Autodesk Inventor part; units mm, degrees
ref_plane "Work Plane3" through (158.3589, -41.348, 102.8428) normal (0, 0, -1) x (-1, 0, 0)
ref_plane "Work Plane5" through (0, -98.2767, 225.7428) normal (0, 1, 0) x (-1, 0, 0)
ref_plane "YZ Plane" through (0, 0, 0) normal (1, 0, 0) x (0, 1, 0)
ref_plane "Work Plane3" through (158.3589, -41.348, 102.8428) normal (0, 0, -1) x (-1, 0, 0)
sketch "Sketch3" plane through (158.3589, -41.348, 102.8428) normal (0, 0, -1) x (-1, 0, 0)
  circle A0 centre (0, 0) radius 10.5
  arc A1 (-3, 10.0623) -> (3, 10.0623) centre (0, 0) ccw
  line L0 (0, 0) -> (0, 16.5106) construction
  line L1 (5, 13.0767) -> (5, 23.0767)
  line L2 (3, 10.0623) -> (3, 23.0767)
  line L3 (5, 23.0767) -> (3, 23.0767)
  line L4 (-5, 13.0767) -> (-5, 23.0767)
  line L5 (-3, 10.0623) -> (-3, 23.0767)
  line L6 (-5, 23.0767) -> (-3, 23.0767)
  arc A2 (-5, 13.0767) -> (5, 13.0767) centre (0, 0) ccw
  point P0 (158.3589, 41.348)
  dimension "d8" = 0
  dimension "d30" = 10
  dimension "d31" = 2
  dimension "d32" = 3
  dimension "d33" = 14
extrude "Extrusion2" add sketch "Sketch3" against normal blind 15 contours A0 L2 L3 L1 A2 L4 L6 L5
sketch "Sketch5" plane through (158.3589, -41.348, 102.8428) normal (0, 0, -1) x (-1, 0, 0)
  line L0 (-41.6411, -56.9287) -> (358.3589, -56.9287)
  arc A0 (-2.5, 13.775) -> (2.5, 13.775) centre (0, 0) ccw
  line L1 (0, -14) -> (0, -56.9287) construction
  line L2 (9, -10.7238) -> (9, -56.9287)
  line L3 (-9, -10.7238) -> (-9, -56.9287)
  point P0 (158.3589, 41.348)
  point P1 (-9, -10.7238)
  point P2 (-9, -56.9287)
  dimension "d19" = 9
extrude "Extrusion4" add sketch "Sketch5" against normal blind 15
ref_plane "Work Plane5" through (0, -98.2767, 225.7428) normal (0, 1, 0) x (-1, 0, 0)
sketch "Sketch7" plane through (0, -98.2767, 225.7428) normal (0, 1, 0) x (-1, 0, 0)
  circle A0 centre (-143.3589, -112.9) radius 2
  circle A1 centre (-173.3589, -112.9) radius 2
  line L0 (-134.3589, -107.9) -> (-182.3589, -107.9)
  line L1 (-182.3589, -107.9) -> (-182.3589, -122.9)
  line L2 (-182.3589, -122.9) -> (-134.3589, -122.9)
  line L3 (-134.3589, -122.9) -> (-134.3589, -107.9)
  line L4 (-144.3589, -107.9) -> (-155.8589, -107.9)
  point P0 (0, -225.7428)
  point P1 (-149.3589, -107.9)
  dimension "d23" = 48
  dimension "d24" = 15
  dimension "d25" = 9
extrude "Extrusion5" add sketch "Sketch7" along normal blind 3
sketch "Sketch8" plane through (153.3589, -28.2713, 102.8428) normal (-1, 0, 0) x (0, 0, 1)
  line L0 (0, 0) -> (0, 10)
  line L1 (0, 10) -> (15, 10)
  line L2 (0, 5) -> (15, 5) construction
  line L3 (0, 10) -> (15, 10)
  line L4 (7.5, 10) -> (7.5, 0) construction
  circle A0 centre (7.5, 5) radius 2
  point P0 (-102.8428, 28.2713)
  dimension "d34" = 4
extrude "Extrusion6" cut sketch "Sketch8" against normal blind 10
properties part number "base_motor"
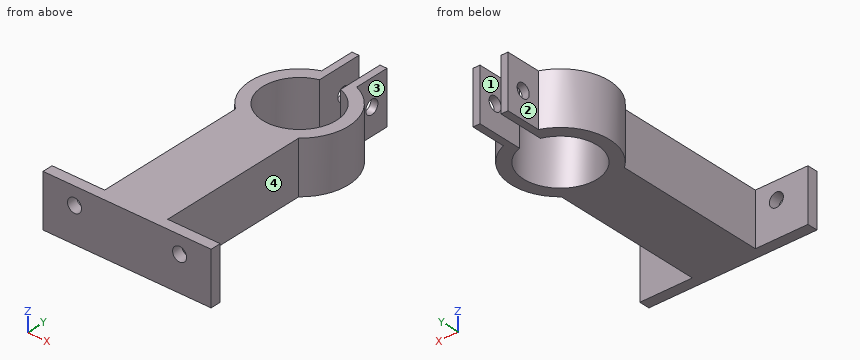
Verification items for the finished model (mm, model axes). Face numbers are marked on the shaded views. A direction names the side the tool comes from. Round coordinates to 2 decimals unless told otherwise and drop trailing zeros. Order: outer loops, then holes, each group sorted by start corner. A loop starts at its lowest first (then second) coordinate and runs counter-clockwise, first axis right, second up. Notation, with made-up numbers: (8.25, 37) -> (21.25, 37) arc R21 cw to (21.25, 68) -> close; hole circle Ø6 at (-36, 45). An arc over 180 degrees is marked (long way). Put each result on its own line as item: value. Start each with the question number.
(1) Section check A-A (x = 165). Enter the section's corners in (y, z) (3 decimals).
(2) Section check D-D (z = 105). Enter the section's corners in (x, y).
(3) Material ranges on line 1 along X through (y, z) = (-28, 111.25); line 2 along X through (y, z) = (-64.5, 104); line 3 along Y through (x, z) = (170, 109.5), recorded low to high.
(4) Section check B-B (z = 110). Enter the section's corners in (x, y), then the cut area to 3 significant figures.
(5) Section check C-C (y = -34). Enter the section's corners in (x, z), then the cut area to 3 significant figures.
(6) Tool access check on the marked faces 1, 2, 3 and 4. Record the directions out of +Z, -Z, +X, -X, +Y, -Y that give a thin tool (end or side, any length) a straight path to the whole face; none if there is none.
(7) Depth check by flat-ended pin: pin 1 Ø4.5 at (x, z) = (175, 111.5) entering from +Y; pin 2 Ø7.5 at (y, z) = (-79.5, 113) entering from -X; pin 3 Ø8 at (y, z) = (-52.5, 114) entering from -X; pin 4 Ø3 at (y, z) = (-23.27, 110.34) entering from -X. Enter the tip coordinate at first touch or a pass-through.
Completed:
1. outline: (-98.277, 102.843) -> (-49.481, 102.843) -> (-49.481, 117.843) -> (-98.277, 117.843) -> close; (-33.215, 102.843) -> (-29.023, 102.843) -> (-29.023, 117.843) -> (-33.215, 117.843) -> close
2. outline: (134.36, -98.28) -> (182.36, -98.28) -> (182.36, -95.28) -> (167.36, -95.28) -> (167.36, -52.07) arc R14 ccw to (163.36, -28.27) -> (163.36, -18.27) -> (161.36, -18.27) -> (161.36, -31.29) arc R10.5 cw (long way) to (155.36, -31.29) -> (155.36, -18.27) -> (153.36, -18.27) -> (153.36, -28.27) arc R14 ccw to (149.36, -52.07) -> (149.36, -95.28) -> (134.36, -95.28) -> close
3. line 1: x = 153.36 to 155.36, 161.36 to 163.36
3. line 2: x = 149.36 to 167.36
3. line 3: y = -98.28 to -95.28, -49.13 to -33.57
4. outline: (134.36, -98.28) -> (182.36, -98.28) -> (182.36, -95.28) -> (167.36, -95.28) -> (167.36, -52.07) arc R14 ccw to (163.36, -28.27) -> (163.36, -25.24) -> (161.36, -25.24) -> (161.36, -31.29) arc R10.5 cw (long way) to (155.36, -31.29) -> (155.36, -25.24) -> (153.36, -25.24) -> (153.36, -28.27) arc R14 ccw to (149.36, -52.07) -> (149.36, -95.28) -> (134.36, -95.28) -> close; (153.36, -21.3) -> (155.36, -21.3) -> (155.36, -18.27) -> (153.36, -18.27) -> close; (161.36, -21.3) -> (163.36, -21.3) -> (163.36, -18.27) -> (161.36, -18.27) -> close
4. area: 1,150 mm2
5. outline: (146.44, 102.84) -> (150.86, 102.84) -> (150.86, 117.84) -> (146.44, 117.84) -> close; (165.86, 102.84) -> (170.28, 102.84) -> (170.28, 117.84) -> (165.86, 117.84) -> close
5. area: 132 mm2
6. face 1: +Z, -Z, +Y
6. face 2: +Z, -Z, -X, +Y
6. face 3: +Z, -Z, +X, +Y
6. face 4: +Z, -Z, +X
7. pin 1: stops at y = -95.28
7. pin 2: stops at x = 149.36
7. pin 3: stops at x = 146.32
7. pin 4: passes through
